Check sheet for the drawn part. Datum: minimum x, y, z corner. Units: mm. A direction names the side the tool comes from. Give positions to 0.01 mm unless a question says otherwise; leave off trailing zeros. Loops run counter-clockwise (first coordinate to the right, second up) from the corner with the lowest first, then second, coordinate; pieces in that order, holes last. Notation, with made-up numbers: (2.25, -0.5) - (52.25, -0.5) arc R17 cw to (52.25, 4.5) - close; hole circle Ø10 at (37, 31). An arc over 180 degrees is marked (long way). Answer in a Markdown table with one row per item.
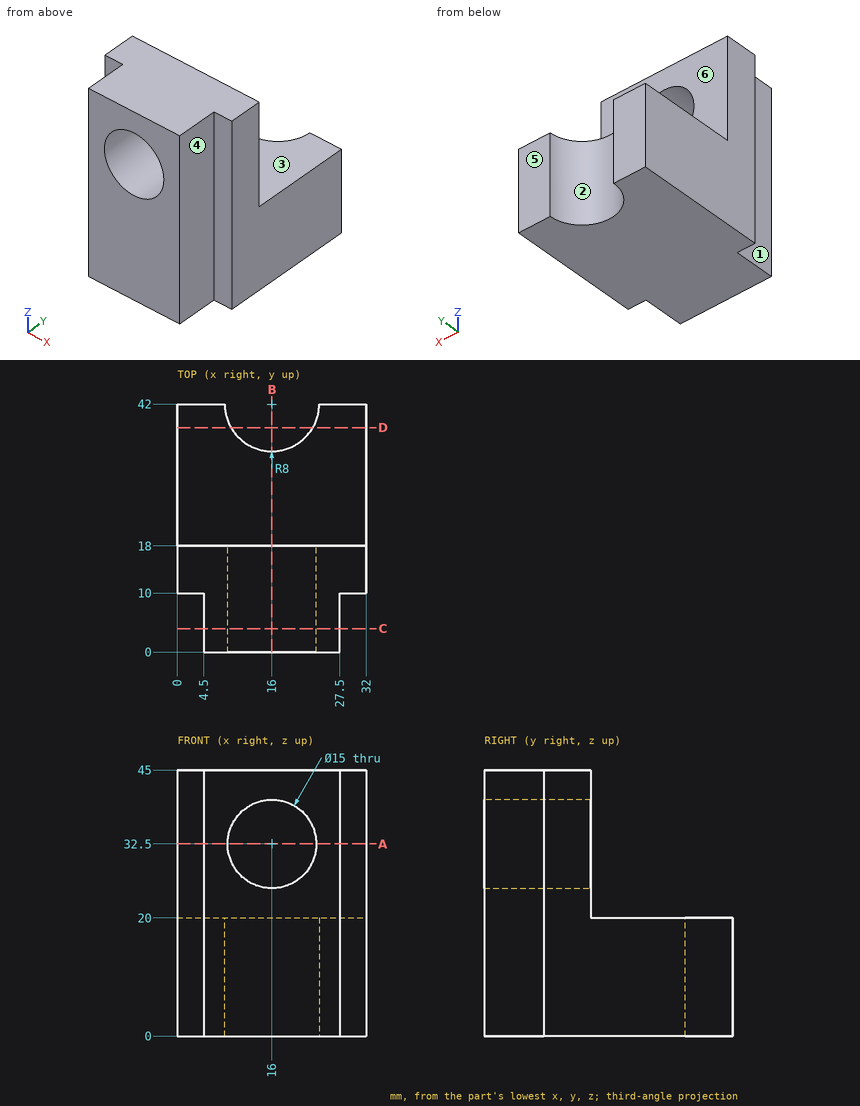
Q1. Sectioned sample at C-C (y = 4). Record the cut outline in (x, z).
Completed:
| item | result |
|---|---|
| outline | (4.5, 0) - (27.5, 0) - (27.5, 45) - (4.5, 45) - close; hole circle Ø15 at (16, 32.5) |
Q2. Sectioned sample at D-D (y = 38). Record the cut outline in (x, z), and give its area (3 significant figures).
Completed:
| item | result |
|---|---|
| outline | (0, 0) - (9.07, 0) - (9.07, 20) - (0, 20) - close; (22.93, 0) - (32, 0) - (32, 20) - (22.93, 20) - close |
| area | 363 mm^2 |
Q3. Draft check along X on the marked faces 1, 2 and 3. Enter one of: +X half, -X half, draft (parallel to the pull), parting line (faces both ways), or undercut.
Completed:
| item | result |
|---|---|
| face 1 | -X half |
| face 2 | undercut |
| face 3 | draft |
Q4. Sectioned sample at A-A (z = 32.5). Record the cut outline in (x, y).
Completed:
| item | result |
|---|---|
| outline | (0, 10) - (4.5, 10) - (4.5, 0) - (8.5, 0) - (8.5, 18) - (0, 18) - close; (23.5, 0) - (27.5, 0) - (27.5, 10) - (32, 10) - (32, 18) - (23.5, 18) - close |
Q5. Tool access check on the marked faces 4, 5 and 6. Record the directions out of +Z, -Z, +X, -X, +Y, -Y that give a thin tool (end or side, any length) a straight path to the whole face; none if there is none.
Completed:
| item | result |
|---|---|
| face 4 | +Z, -Z, +X, -Y |
| face 5 | +Z, -Z, +X, -X, +Y |
| face 6 | +Z, +X, -X, +Y |
Q6. Go/stop test with flat-tipped pins: P1, Ø3.5, axis at x = 29.5, z = 22.5, coming from the -Y side; P2, Ø11, axis at y = 3, z = 16.5, coming from the -X side; P3, Ø4, axis at x = 11, y = 33, coming from the +Z side. Record where each tip stops, or that it passes through.
Completed:
| item | result |
|---|---|
| P1 | y = 10 |
| P2 | x = 4.5 |
| P3 | z = 20 |
Q7. Thickness scan on line 1 (X direction, y = 13.75, z = 32.5); line 2 (X direction, y = 3, z = 11); line 3 (Y direction, x = 16, z = 24.5). Record the ranges inside material, lowest first.
Completed:
| item | result |
|---|---|
| line 1 | 0 to 8.5, 23.5 to 32 |
| line 2 | 4.5 to 27.5 |
| line 3 | 0 to 18 |
Q8. Sectioned sample at B-B (x = 16). Record the cut outline in (y, z).
Completed:
| item | result |
|---|---|
| outline | (0, 0) - (34, 0) - (34, 20) - (18, 20) - (18, 25) - (0, 25) - close; (0, 40) - (18, 40) - (18, 45) - (0, 45) - close |
